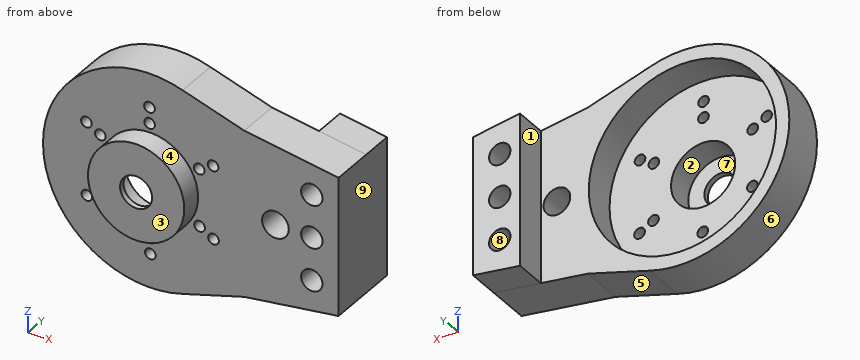
Autodesk Inventor part; units mm, degrees
ref_plane "YZ Plane" through (0, 0, 0) normal (1, 0, 0) x (0, 1, 0)
ref_plane "XZ Plane" through (0, 0, 0) normal (0, 1, 0) x (-1, 0, 0)
ref_plane "XY Plane" through (0, 0, 0) normal (0, 0, 1) x (1, 0, 0)
sketch "Эскиз1" plane through (0, 0, 0) normal (0, 1, 0) x (-1, 0, 0)
  arc A0 (13.2517, 5.1196) -> (11.6396, 8.8847) centre (11.8859, 6.7625) ccw
  line L0 (11.6396, 8.8847) -> (3.5765, 5.9707)
  line L1 (3.5765, 5.9707) -> (2.1921, 14.0362)
  arc A1 (2.1921, 14.0362) -> (-1.8746, 14.5225) centre (0.0865, 13.6747) ccw
  line L2 (-1.8746, 14.5225) -> (-3.3825, 6.0827)
  line L3 (-3.3825, 6.0827) -> (-11.0596, 8.9165)
  arc A2 (-11.0596, 8.9165) -> (-13.5142, 5.6378) centre (-11.7994, 6.9122) ccw
  line L4 (-13.5142, 5.6378) -> (-6.959, 0.112)
  line L5 (-6.959, 0.112) -> (-13.2517, -5.1196)
  arc A3 (-13.2517, -5.1196) -> (-11.6396, -8.8847) centre (-11.8859, -6.7625) ccw
  line L6 (-11.6396, -8.8847) -> (-3.5765, -5.9707)
  line L7 (-3.5765, -5.9707) -> (-2.1921, -14.0362)
  arc A4 (-2.1921, -14.0362) -> (1.8746, -14.5225) centre (-0.0865, -13.6747) ccw
  line L8 (1.8746, -14.5225) -> (3.3825, -6.0827)
  line L9 (3.3825, -6.0827) -> (11.0596, -8.9165)
  arc A5 (11.0596, -8.9165) -> (13.5142, -5.6378) centre (11.7994, -6.9122) ccw
  line L10 (13.5142, -5.6378) -> (6.959, -0.112)
  line L11 (6.959, -0.112) -> (13.2517, 5.1196)
  circle A6 centre (6.6709, 3.7954) radius 1
  circle A7 centre (11.8859, 6.7625) radius 1
  circle A8 centre (9.2109, -5.3958) radius 1
  circle A9 centre (-0.0485, -7.6748) radius 1
  circle A10 centre (-0.0865, -13.6747) radius 1
  circle A11 centre (-9.2784, -5.2789) radius 1
  circle A12 centre (-6.6223, 3.8794) radius 1
  circle A13 centre (-11.7994, 6.9122) radius 1
  circle A14 centre (0.0675, 10.6748) radius 1
  circle A15 centre (0, 0) radius 4.75
  circle A16 centre (0.0865, 13.6747) radius 1
  circle A17 centre (0.0485, 7.6748) radius 1
  circle A18 centre (-9.2109, 5.3958) radius 1
  circle A19 centre (-11.8859, -6.7625) radius 1
  circle A20 centre (-6.6709, -3.7954) radius 1
  circle A21 centre (-0.0675, -10.6748) radius 1
  circle A22 centre (11.7994, -6.9122) radius 1
  circle A23 centre (6.6223, -3.8794) radius 1
  circle A24 centre (9.2784, 5.2789) radius 1
  circle A25 centre (0, 0) radius 1.875
  circle A26 centre (0, 0) radius 20
  circle A27 centre (0, 0) radius 17.5
  point P0 (0, 0)
  dimension "d0" = 40
  dimension "d1" = 35
extrude "Выдавливание1" add sketch "Эскиз1" along normal blind 2 contours L11 L10 A5 L9 L8 A4 L7 L6 A3 L5 L4 A2 L3 L2 A1 L1 L0 A0 | A26 | A27
sketch "Эскиз2" plane through (0, 2, 0) normal (0, 1, 0) x (1, 0, 0)
  arc A0 (13.2517, 5.1196) -> (11.6396, 8.8847) centre (11.8859, 6.7625) ccw
  line L0 (11.6396, 8.8847) -> (3.5765, 5.9707)
  line L1 (3.5765, 5.9707) -> (2.1921, 14.0362)
  arc A1 (2.1921, 14.0362) -> (-1.8746, 14.5225) centre (0.0865, 13.6747) ccw
  line L2 (-1.8746, 14.5225) -> (-3.3825, 6.0827)
  line L3 (-3.3825, 6.0827) -> (-11.0596, 8.9165)
  arc A2 (-11.0596, 8.9165) -> (-13.5142, 5.6378) centre (-11.7994, 6.9122) ccw
  line L4 (-13.5142, 5.6378) -> (-6.959, 0.112)
  line L5 (-6.959, 0.112) -> (-13.2517, -5.1196)
  arc A3 (-13.2517, -5.1196) -> (-11.6396, -8.8847) centre (-11.8859, -6.7625) ccw
  line L6 (-11.6396, -8.8847) -> (-3.5765, -5.9707)
  line L7 (-3.5765, -5.9707) -> (-2.1921, -14.0362)
  arc A4 (-2.1921, -14.0362) -> (1.8746, -14.5225) centre (-0.0865, -13.6747) ccw
  line L8 (1.8746, -14.5225) -> (3.3825, -6.0827)
  line L9 (3.3825, -6.0827) -> (11.0596, -8.9165)
  arc A5 (11.0596, -8.9165) -> (13.5142, -5.6378) centre (11.7994, -6.9122) ccw
  line L10 (13.5142, -5.6378) -> (6.959, -0.112)
  line L11 (6.959, -0.112) -> (13.2517, 5.1196)
  circle A6 centre (6.6709, 3.7954) radius 1
  circle A7 centre (11.8859, 6.7625) radius 1
  circle A8 centre (9.2109, -5.3958) radius 1
  circle A9 centre (-0.0485, -7.6748) radius 1
  circle A10 centre (-0.0865, -13.6747) radius 1
  circle A11 centre (-9.2784, -5.2789) radius 1
  circle A12 centre (-6.6223, 3.8794) radius 1
  circle A13 centre (-11.7994, 6.9122) radius 1
  circle A14 centre (0.0675, 10.6748) radius 1
  circle A15 centre (0, 0) radius 4.75
  circle A16 centre (0.0865, 13.6747) radius 1
  circle A17 centre (0.0485, 7.6748) radius 1
  circle A18 centre (-9.2109, 5.3958) radius 1
  circle A19 centre (-11.8859, -6.7625) radius 1
  circle A20 centre (-6.6709, -3.7954) radius 1
  circle A21 centre (-0.0675, -10.6748) radius 1
  circle A22 centre (11.7994, -6.9122) radius 1
  circle A23 centre (6.6223, -3.8794) radius 1
  circle A24 centre (9.2784, 5.2789) radius 1
  circle A25 centre (0, 0) radius 1.875
  circle A26 centre (0, 0) radius 20
  circle A27 centre (0, 0) radius 17.5
  point P0 (0, 0)
  dimension "d4" = 40
  dimension "d5" = 35
extrude "Выдавливание2" add sketch "Эскиз2" along normal blind 6 contours A26
sketch "Эскиз3" plane through (0, 0, 0) normal (0, -1, 0) x (1, 0, 0)
  circle A0 centre (0, 0) radius 20
  line L0 (15.264, 12.9232) -> (15.264, -12.9232)
  line L1 (15.264, 12.9232) -> (35.264, 12.9232)
  line L2 (35.264, 12.9232) -> (35.264, -12.9232)
  line L3 (35.264, -12.9232) -> (15.264, -12.9232)
  line L4 (15.264, -12.9232) -> (15.264, 12.9232)
  dimension "d8" = 20
extrude "Выдавливание3" add sketch "Эскиз3" against normal up to surface (8 mm away) contours A0 L1 L2 L3
sketch "Эскиз4" plane through (0, 0, 0) normal (0, -1, 0) x (1, 0, 0)
  line L0 (35.264, 0) -> (30.264, 0)
  circle A0 centre (30.264, 0) radius 2
  point P0 (0, 0)
  dimension "d17" = 5
  dimension "d18" = 4
extrude "Выдавливание4" cut sketch "Эскиз4" against normal through all
pattern_linear "Прямоуг.массив2" count 3 spacing 8 along (0, 0, 1) of "Выдавливание4" first direction both ways yes
chamfer "Фаска3" distance 11 angle 45 2 edges at (15.264, 4, -12.9232) (15.264, 4, 12.9232)
chamfer "Фаска4" distance 9 angle 45 2 edges at (26.264, 4, 12.9232) (26.264, 4, -12.9232)
sketch "Эскиз8" plane through (0, 8, 0) normal (0, 1, 0) x (1, 0, 0)
  line L0 (17.6524, 15.5384) -> (35.264, 12.9232)
  line L1 (35.264, 12.9232) -> (35.264, -12.9232)
  line L2 (35.264, -12.9232) -> (17.6524, -15.5384)
  line L3 (35.264, 12.9232) -> (17.6524, 15.5384)
  line L4 (26.4582, 14.2308) -> (26.4582, -14.2308)
  line L5 (17.6524, -15.5384) -> (35.264, -12.9232)
  circle A0 centre (30.264, 8) radius 2
  circle A1 centre (30.264, 0) radius 2
  circle A2 centre (30.264, -8) radius 2
  point P0 (0, 0)
extrude "Выдавливание8" add sketch "Эскиз8" along normal blind 6
sketch "Эскиз9" plane through (0, 2, 0) normal (0, 1, 0) x (1, 0, 0)
  circle A0 centre (0, 0) radius 9
  dimension "d44" = 18
extrude "Выдавливание9" add sketch "Эскиз9" against normal blind 6
sketch "Эскиз10" plane through (0, 2, 0) normal (0, 1, 0) x (1, 0, 0)
  circle A0 centre (0, 0) radius 3
  dimension "d48" = 6
extrude "Выдавливание10" cut sketch "Эскиз10" against normal through all
sketch "Эскиз11" plane through (0, 2, 0) normal (0, 1, 0) x (1, 0, 0)
  circle A0 centre (0, 0) radius 6
  dimension "d52" = 12
extrude "Выдавливание11" cut sketch "Эскиз11" against normal blind 5
sketch "Эскиз12" plane through (0, 8, 0) normal (0, 1, 0) x (1, 0, 0)
  line L0 (26.4582, 14.2308) -> (26.4582, -14.2308)
  line L1 (26.4582, 0) -> (23.4582, 0)
  circle A0 centre (23.4582, 0) radius 2.5
  point P0 (0, 0)
  dimension "d56" = 3
  dimension "d57" = 5
extrude "Выдавливание12" cut sketch "Эскиз12" against normal through all
properties part number "000.403 - Рычаг" material "Пластик АБС"
Input: part model. Units: mm. Frame: model coordinates. Face numbers are marked on the shaded views. A direction names the side the tool comes from. Coordinates: 2 decimals unless noted, no trailing zeros. Write each loop counter-clockwise with the first axis right and the second up, starting at its lowest first coordinate (ties: lowest second). Pieces come first, ordered by that corner, then holes.
1) Pin query (flat end, axial travel): pin 1 Ø6 at (y, z) = (5.5, -15.5) entering from -X; pin 2 Ø4 at (x, z) = (23.46, 0) entering from +Y; pin 3 Ø1.5 at (x, z) = (-12.5, 5) entering from +Y; pin 4 Ø2.5 at (x, z) = (-9.28, 5.28) entering from -Y. Return the tip coordinate at first contact, or that it passes through.
2) Section C-C on y = -0.75. Output: boundary loops of the cut face in (x, z).
3) Section A-A on y = 10.25. Output: boundary loops of the cut face in (x, z).
4) Material intervals for line 1 along X through (y, z) = (4.5, 0); line 2 along Z through (x, y) = (0, -0.05); line 3 along Z through (x, y) = (30.5, 1.25), sorted ascending.
5) Set-up query: the marked faces 1, 2, 3, 4 and 5. Return all of +Z, -Z, +X, -X, +Y, -Y with unobstructed straight access to the full face (end or side cutting, diameter ignored); none if empty.
6) Section B-B on z = 0. State how many separate pieces and enclosed holes the cut face has, and give its area (3 significant figures).
7) Mould query, pull axis X, two halves, no side actions, for the marked faces 6, 7, 8 and 9. Classes: pulls with the +X half, pulls with the -X half, needs draft (parallel to the pull), parting line crosses it, or undercut.
Check result:
1. pin 1: stops at x = -15.61
1. pin 2: passes through
1. pin 3: stops at y = 2
1. pin 4: stops at y = 0
2. outline: circle Ø18 at (0, 0); hole circle Ø12 at (0, 0)
3. outline: (26.46, -14.23) - (35.26, -12.92) - (35.26, 12.92) - (26.46, 14.23) - close; hole circle Ø4 at (30.26, -8); hole circle Ø4 at (30.26, 0); hole circle Ø4 at (30.26, 8)
4. line 1: x = -20 to -17.5, 17.5 to 20.96, 25.96 to 28.26, 32.26 to 35.26
4. line 2: z = -9 to -6, 6 to 9
4. line 3: z = -13.63 to -9.99, -6.01 to -1.99, 1.99 to 6.01, 9.99 to 13.63
5. face 1: +Z, -Z, -X, +Y
5. face 2: +Y
5. face 3: +Z, -Z, +X, -X, -Y
5. face 4: -Y
5. face 5: -Z, +X, +Y, -Y
6. separate pieces: 4
6. enclosed holes: 0
6. area: 195 mm2
7. face 6: parting line crosses it
7. face 7: undercut
7. face 8: undercut
7. face 9: pulls with the +X half
